Answer from the drawing. Dimensions are ordinates in mm from the lowest x, y and z of the part. Give positions to 0.01 mm unless a question says otherwise; leave off trailing zeros. Write each loop counter-clockwise with the first axis right and the second up, starting at its lowest first coordinate (ties: lowest second). Pieces come first, ordered by that corner, then holes.
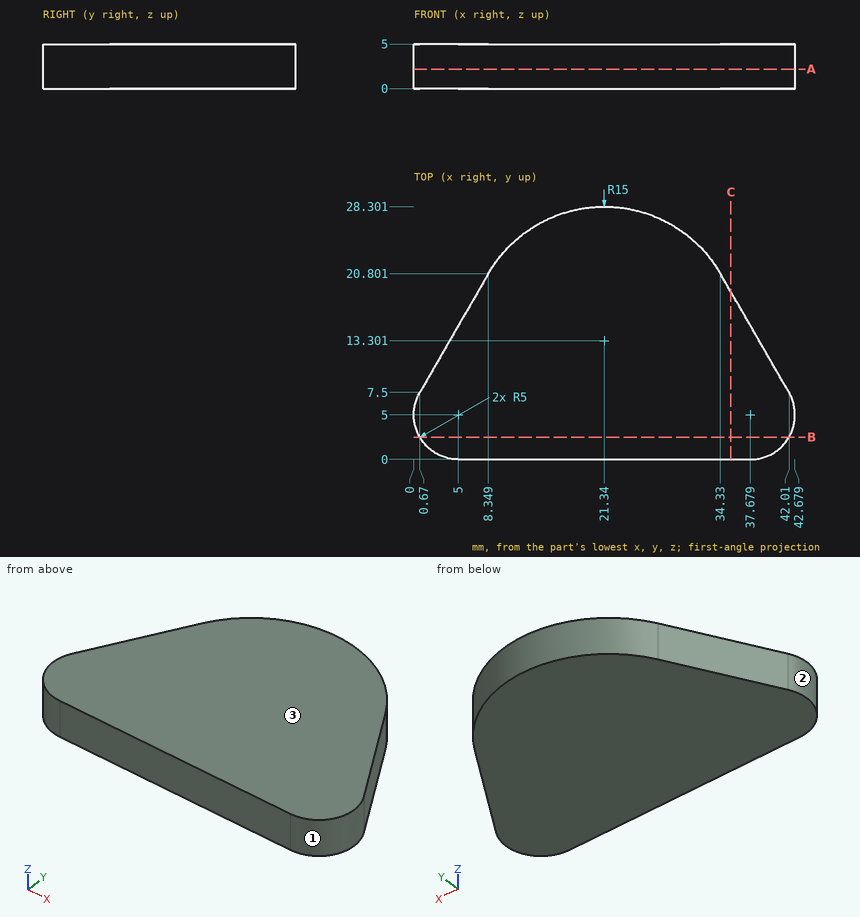
Item 1: Section A-A (z = 2.2) is taken. Write down the section's boundary in (x, y), and give its area (3 significant figures).
Result set:
outline: (0.67, 7.5) arc R5 ccw to (5, 0) - (37.68, 0) arc R5 ccw to (42.01, 7.5) - (34.33, 20.8) arc R15 ccw to (8.35, 20.8) - close
area: 894 mm2
Item 2: Determine the mould class of the marked faces 1, 2 and 3 for opening direction X: pulls with the +X half, pulls with the -X half, needs draft (parallel to the pull), parting line crosses it, or undercut.
Result set:
face 1: pulls with the +X half
face 2: pulls with the -X half
face 3: needs draft
Item 3: Section C-C (x = 35.5) is taken. Write down the section's boundary in (y, z) (1 decimal).
Result set:
outline: (0, 0) - (18.8, 0) - (18.8, 5) - (0, 5) - close
Item 4: This flat-tipped pin is pushed along its axis until it touches: pin 1 Ø3 at (y, z) = (14.5, 3) entering from +X (1 decimal). Where does it stop, or does it pass through?
Result set:
pin 1: stops at x = 38.8
Item 5: Section B-B (y = 2.5) is taken. Write down the section's boundary in (x, z).
Result set:
outline: (0.67, 0) - (42.01, 0) - (42.01, 5) - (0.67, 5) - close
Item 6: Find the intervals of material crossed by line 1 along Y through (x, z) = (21, 2.9); line 2 along Y through (x, z) = (38.5, 3.8) (1 decimal); line 3 along X through (y, z) = (10.25, 4.8), in increasing order.
Result set:
line 1: y = 0 to 28.3
line 2: y = 0.1 to 13.6
line 3: x = 2.26 to 40.42
